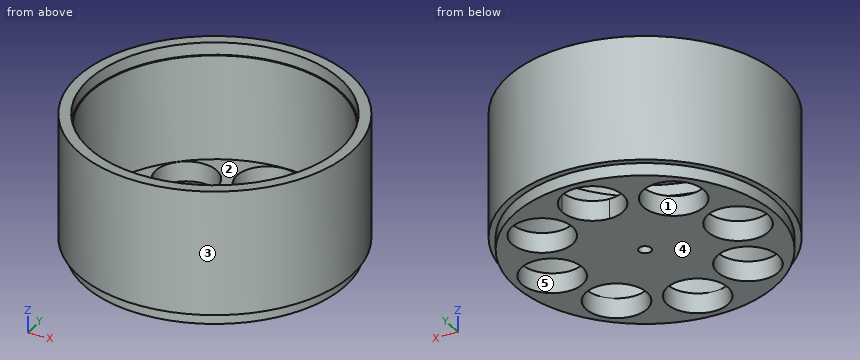
from build123d import *

# Parameters (mm, degrees)
F0_R        = 52.5
F0_R_2      = 2.5
F1_DEPTH    = 5
F0_R_3      = 55
F1_FACE_R   = 52.5
F1_FACE_R_2 = 2.5
F2_DEPTH    = 50
F3_R        = 50
F3_R_2      = 2.5
F4_DEPTH    = 47
F5_R        = 12.25
F6_DEPTH    = 8
F7_R        = 50.5
F7_R_2      = 50
F8_DEPTH    = 5


with BuildPart() as f1:
    # F0 (on Top) → F1 (new body)
    with BuildSketch(Plane.XY):
        Circle(F0_R)
        Circle(F0_R_2, mode=Mode.SUBTRACT)
    extrude(amount=-F1_DEPTH)

    # F0 (on Top) + F1_face (on face) → F2 (join)
    with BuildSketch(Plane.XY):
        Circle(F0_R_3)
        Circle(F0_R, mode=Mode.SUBTRACT)
    with BuildSketch(Plane.XY):
        Circle(F1_FACE_R)
        Circle(F1_FACE_R_2, mode=Mode.SUBTRACT)
    extrude(amount=F2_DEPTH)

    # F3 (on face) → F4 (cut)
    with BuildSketch(Plane.XY.offset(50)):
        Circle(F3_R)
        Circle(F3_R_2, mode=Mode.SUBTRACT)
    extrude(amount=-F4_DEPTH, mode=Mode.SUBTRACT)

    # F5 (on face) → F6 (cut)
    with BuildSketch(Plane.XY.offset(3)):
        with BuildLine():
            ThreePointArc((0, 25.25), (8.662058, 28.837942), (12.25, 37.5))
            ThreePointArc((12.25, 37.5), (-8.662058, 46.162058), (0, 25.25))
        make_face()
        with Locations((-26.516504, 26.516504)):
            Circle(F5_R)
        with Locations((-37.5, 0)):
            Circle(F5_R)
        with Locations((-26.516504, -26.516504)):
            Circle(F5_R)
        with Locations((0, -37.5)):
            Circle(F5_R)
        with Locations((26.516504, -26.516504)):
            Circle(F5_R)
        with Locations((26.516504, 26.516504)):
            Circle(F5_R)
        with Locations((37.5, 0)):
            Circle(F5_R)
    extrude(amount=-F6_DEPTH, mode=Mode.SUBTRACT)

    # F7 (on face) → F8 (cut)
    with BuildSketch(Plane.XY.offset(50)):
        Circle(F7_R)
        Circle(F7_R_2, mode=Mode.SUBTRACT)
    extrude(amount=-F8_DEPTH, mode=Mode.SUBTRACT)


solid = f1.part
Input: part model. Units: mm. Frame: model coordinates. Face numbers are marked on the shaded views. A direction names the side the tool comes from. Round coordinates to 2 decimals unless told otherwise and drop trailing zeros. Write each loop counter-clockwise with the first axis right and the second up, starting at its lowest first coordinate (ties: lowest second). Pieces come first, ordered by that corner, then holes.
1) Cut plane C-C (x = -35.5). Return the cut outline in (y, z).
2) Cut plane B-B (z = 39). Return the cut outline in (x, y), then the cut area to 3 significant figures.
3) Reachability of the marked faces 1 and 2 from +Z, -Z, +X, -X, +Y, -Y: full face, straight path, thin tool, end or side. Return the list, or none.
4) Contact query for flat-ended pins moving along their axis: P1, Ø12, axis at x = 25, z = 13, coming from the +Y side; P2, Ø10, axis at x = 9, z = 23.5, coming from the +Y side; P3, Ø12, axis at y = 29.5, z = 39.5, coming from the -X side. Output: stop coordinate, or through.
5) Ray query, L1, parallel to Y at x = 0, z = 1.25; L2, parallel to Y at x = -1, z = 31.5; L3, parallel to X at y = -7, z = -2. Return the intervals inside material, ascending.
6) Draft query along X for the marked faces 3, 4 and 5. Return one class per face: pulls with the +X half, pulls with the -X half, needs draft (parallel to the pull), parting line crosses it, or undercut.
7) Cut plane A-A (y = 0). Return the cut outline in (x, z), then the cut area to 3 significant figures.
Geometry says:
1. outline: (-42.01, 0) - (-38.68, 0) - (-38.68, -5) - (-34.84, -5) - (-34.84, 3) - (-35.21, 3) - (-35.21, 45) - (-35.92, 45) - (-35.92, 50) - (-42.01, 50) - close; (-18.19, -5) - (-12.09, -5) - (-12.09, 3) - (-18.19, 3) - close; (12.09, -5) - (18.19, -5) - (18.19, 3) - (12.09, 3) - close; (34.84, -5) - (38.68, -5) - (38.68, 0) - (42.01, 0) - (42.01, 50) - (35.92, 50) - (35.92, 45) - (35.21, 45) - (35.21, 3) - (34.84, 3) - close
2. outline: circle Ø110 at (0, 0); hole circle Ø100 at (0, 0)
2. area: 1,650 mm2
3. face 1: +Z, -Z
3. face 2: +Z
4. P1: stops at y = 51.61
4. P2: stops at y = 54.85
4. P3: stops at x = -49.73
5. L1: y = -55 to -49.75, -25.25 to -2.5, 2.5 to 25.25, 49.75 to 55
5. L2: y = -54.99 to -49.99, 49.99 to 54.99
5. L3: x = -52.03 to -47.55, -27.45 to 27.45, 47.55 to 52.03
6. face 3: parting line crosses it
6. face 4: needs draft
6. face 5: undercut
7. outline: (-55, 0) - (-52.5, 0) - (-52.5, -5) - (-49.75, -5) - (-49.75, 3) - (-50, 3) - (-50, 45) - (-50.5, 45) - (-50.5, 50) - (-55, 50) - close; (-25.25, -5) - (-2.5, -5) - (-2.5, 3) - (-25.25, 3) - close; (2.5, -5) - (25.25, -5) - (25.25, 3) - (2.5, 3) - close; (49.75, -5) - (52.5, -5) - (52.5, 0) - (55, 0) - (55, 50) - (50.5, 50) - (50.5, 45) - (50, 45) - (50, 3) - (49.75, 3) - close
7. area: 888 mm2
